from build123d import *

# Parameters (mm, degrees)
SKETCH_R   = 4.064
BODY_DEPTH = 6.1
SKETCH1_R  = 0.5
LEGS_DEPTH = 10
LIP_DEPTH  = 0.5
FILLET2_R  = 0.5


with BuildPart() as part:
    # sketch → Body (new body)
    with BuildSketch(Plane(origin=(0, 4.06, 0), x_dir=(1, 0, 0), z_dir=(0, 1, 0))):
        with Locations((-2.54, 0)):
            Circle(SKETCH_R)
    extrude(amount=BODY_DEPTH)

    # Sketch1 → Legs (add)
    with BuildSketch(Plane.XZ.offset(-4.06)):
        Circle(SKETCH1_R)
        with Locations((-2.54, -2.54)):
            Circle(SKETCH1_R)
        with Locations((-5.08, 0)):
            Circle(SKETCH1_R)
    extrude(amount=LEGS_DEPTH)

    # Sketch3 → Lip (add)
    with BuildSketch(Plane.XZ.offset(-4.06)):
        with BuildLine():
            Line((1.236134349, 4.48324113), (1.94324113, 3.776134349))
            Line((1.94324113, 3.776134349), (1.377555705, 3.210448924))
            ThreePointArc((1.377555705, 3.210448924), (-6.121495847, -3.581495847), (0.670448924, 3.917555705))
            Line((0.670448924, 3.917555705), (1.236134349, 4.48324113))
        make_face()
    extrude(amount=-LIP_DEPTH)

    # Fillet2
    fillet2_edges = [part.edges().sort_by_distance(p)[0] for p in [
        (-6.604, 4.56, 0),
        (-6.604, 10.16, 0),
    ]]
    fillet(fillet2_edges, radius=FILLET2_R)


solid = part.part
Build history of the part. All positions in model axes, mm. A direction names the side the tool comes from. Coordinates: 2 decimals unless noted, no trailing zeros. Order: outer loops, then holes, each group sorted by start corner. A loop starts at its lowest first (then second) coordinate and runs counter-clockwise, first axis right, second up. Notation, with made-up numbers: (49, 40.25) -> (98, 40.25) arc R21 cw to (98, 77.25) -> close; hole circle Ø7 at (29, -26). An arc over 180 degrees is marked (long way). One line per item, written item: value.
(1) Probe line 1 (Y direction, x = 0.75, z = 0.75); line 2 (Y direction, x = 1.5, z = 3.5); line 3 (X direction, y = 4.25, z = -0.5). List the from-to ranges inside material, lowest first. Write a range as [from, to].
Checked values:
line 1: [4.06, 10.16]
line 2: [4.06, 4.56]
line 3: [-7.58, 2.5]
(2) Mould opens along X. For faces 1 (the cylindrical face through (-0.108, -0.87, -0.488)), 2 (the flat face through (-3, 10.16, 0)), 3 (the cylindrical face through (-2.909, -0.87, -2.202)) say: pulls with the +X half, pulls with the -X half, needs draft (parallel to the pull), parting line crosses it, or undercut.
Checked values:
face 1: undercut
face 2: needs draft
face 3: parting line crosses it
(3) Drop flat-ended pins along their axis: pin 1 Ø1 at (x, y) = (0, -1.5) entering from -Z; pin 2 Ø4 at (x, y) = (1.5, -0.5) entering from +Z; pin 3 Ø1.5 at (x, z) = (1, -1) entering from +Y; pin 4 Ø2 at (x, y) = (-3, 2) entering from -Z. Give the stop position or say it passes through.
Checked values:
pin 1: z = -0.5
pin 2: z = 0.5
pin 3: y = 10.16
pin 4: z = -3.04
(4) Tool access for faces 4 (the cylindrical face through (-6, 4.3, -3.7)), 5 (the cylindrical face through (-0.665, 7.328, 3.605)), 6 (the cylindrical face through (-5.58, -0.87, 0.02)): list every direction of +Z, -Z, +X, -X, +Y, -Y with a clear straight run to the whole face (end or side of a thin tool).
Checked values:
face 4: +Y, -Y
face 5: +Y
face 6: -Y
(5) Slice it at B-B, the plane z = 0. List the corners of the cut face in (x, y) (3 decimals).
Checked values:
outline: (-7.605, 4.06) -> (-5.58, 4.06) -> (-5.58, -5.94) -> (-4.58, -5.94) -> (-4.58, 4.06) -> (-0.5, 4.06) -> (-0.5, -5.94) -> (0.5, -5.94) -> (0.5, 4.06) -> (2.525, 4.06) -> (2.525, 4.56) -> (2.024, 4.56) arc R0.5 cw to (1.524, 5.06) -> (1.524, 9.66) arc R0.5 ccw to (1.024, 10.16) -> (-6.104, 10.16) arc R0.5 ccw to (-6.604, 9.66) -> (-6.604, 5.06) arc R0.5 cw to (-7.104, 4.56) -> (-7.605, 4.56) -> close
(6) Slice it at A-A, the plane x = -2.54. List the corners of the cut face in (y, z) (3 decimals), plus the area to 3 significant figures.
Checked values:
outline: (-5.94, -3.04) -> (4.06, -3.04) -> (4.06, -5.065) -> (4.56, -5.065) -> (4.56, -4.564) arc R0.5 cw to (5.06, -4.064) -> (9.66, -4.064) arc R0.5 ccw to (10.16, -3.564) -> (10.16, 3.564) arc R0.5 ccw to (9.66, 4.064) -> (5.06, 4.064) arc R0.5 cw to (4.56, 4.564) -> (4.56, 5.065) -> (4.06, 5.065) -> (4.06, -2.04) -> (-5.94, -2.04) -> close
area: 60.6 mm2
(7) Slice it at C-C, the plane y = -2.5. List the corners of the cut face in (x, z), plus the area to 3 significant figures.
Checked values:
outline: circle Ø1 at (-5.08, 0); circle Ø1 at (-2.54, -2.54); circle Ø1 at (0, 0)
area: 2.36 mm2
